CAD build for the part. Positions are in the model's coordinates, mm. A direction names the side the tool comes from. Give positions to 0.01 mm unless a question says otherwise; leave off trailing zeros. Write each loop counter-clockwise with the first axis right and the second up, starting at its lowest first coordinate (ties: lowest second). Pieces come first, ordered by that corner, then holes. Notation, with made-up numbers: (33.5, 45) -> (79.5, 45) arc R15 ccw to (79.5, 57) -> close; hole circle Ø10 at (55, 63.5). An arc over 180 degrees is marked (long way). Use one line per item in the form item = value. Start each with the question number.
Autodesk Inventor part; units mm, degrees
ref_plane "Work Plane1" through (0, 0, 10) normal (0, 0, 1) x (1, 0, 0)
ref_plane "YZ Plane" through (0, 0, 0) normal (1, 0, 0) x (0, 1, 0)
ref_plane "XZ Plane" through (0, 0, 0) normal (0, 1, 0) x (-1, 0, 0)
ref_plane "Work Plane1" through (0, 0, 10) normal (0, 0, 1) x (1, 0, 0)
sketch "Sketch1" plane through (0, 0, 10) normal (0, 0, 1) x (1, 0, 0)
  line L0 (-4.0299, -0.3538) -> (-2.2322, 1.4439) construction
  arc A0 (-1.4439, 2.2322) -> (-2.2322, 1.4439) centre (-0.9299, 0.9299) ccw construction
  line L1 (-1.4439, 2.2322) -> (0.3538, 4.0299) construction
  line L2 (-37.8299, 42.8299) -> (-37.8299, 37.8299) construction
  line L3 (-37.8299, 37.8299) -> (-42.9208, 37.8299) construction
  line L4 (-37.8299, 42.2137) -> (-37.8299, 45.8299) construction
  line L5 (-37.8299, 45.8299) -> (-4.0299, 45.8299) construction
  line L6 (-4.0299, 45.8299) -> (-4.0299, 42.2137) construction
  line L7 (-4.0299, 4.0299) -> (0.3538, 4.0299)
  circle A1 centre (-20.9299, 20.9299) radius 17.5
  line L8 (-20.9299, 58.9723) -> (17.1124, 20.9299) construction
  line L9 (17.1124, 20.9299) -> (-20.9299, -17.1124) construction
  line L10 (-20.9299, -17.1124) -> (-58.9723, 20.9299) construction
  line L11 (-58.9723, 20.9299) -> (-20.9299, 58.9723) construction
  line L12 (-20.9299, 58.9723) -> (-20.9299, -17.1124) construction
  line L13 (17.1124, 20.9299) -> (-58.9723, 20.9299) construction
  line L14 (-20.9299, 58.9723) -> (32.8701, 58.9723) construction
  line L15 (-43.4299, 43.4299) -> (1.5701, 43.4299) construction
  line L16 (1.5701, 43.4299) -> (1.5701, -1.5701) construction
  line L17 (1.5701, -1.5701) -> (-43.4299, -1.5701) construction
  line L18 (-43.4299, -1.5701) -> (-43.4299, 43.4299) construction
  line L19 (-43.4299, 43.4299) -> (1.5701, -1.5701) construction
  line L20 (1.5701, 43.4299) -> (-43.4299, -1.5701) construction
  line L21 (-43.4299, 5.3876) -> (-43.4299, 36.4723)
  line L22 (-43.4299, 36.4723) -> (-36.4723, 43.4299)
  line L23 (-36.4723, 43.4299) -> (-5.3876, 43.4299)
  line L24 (-5.3876, 43.4299) -> (1.5701, 36.4723)
  line L25 (1.5701, 36.4723) -> (1.5701, 5.3876)
  line L26 (1.5701, 5.3876) -> (-5.3876, -1.5701)
  line L27 (-5.3876, -1.5701) -> (-36.4723, -1.5701)
  line L28 (-36.4723, -1.5701) -> (-43.4299, 5.3876)
  line L29 (-4.0299, 42.2137) -> (-37.8299, 42.2137)
  line L30 (-4.0299, -0.3538) -> (-4.0299, 4.0299)
  circle A2 centre (-20.9299, 20.9299) radius 1.5
  line L31 (-10.9299, 10.9299) -> (-30.9299, 10.9299) construction
  line L32 (-30.9299, 10.9299) -> (-30.9299, 30.9299) construction
  line L33 (-30.9299, 30.9299) -> (-10.9299, 30.9299) construction
  line L34 (-10.9299, 30.9299) -> (-10.9299, 10.9299) construction
  line L35 (-10.9299, 10.9299) -> (-30.9299, 30.9299) construction
  line L36 (-30.9299, 10.9299) -> (-10.9299, 30.9299) construction
  circle A3 centre (-30.9299, 30.9299) radius 1.4
  circle A4 centre (-30.9299, 10.9299) radius 1.4
  circle A5 centre (-10.9299, 10.9299) radius 1.4
  line L37 (-45.8299, 37.8299) -> (-42.0723, 37.8299) construction
  line L38 (-42.1723, 37.7299) -> (-45.8299, 37.7299)
  line L39 (-45.8299, 37.7299) -> (-45.8299, 4.1299)
  line L40 (-45.8299, 4.1299) -> (-42.1723, 4.1299)
  line L41 (-42.1723, 4.1299) -> (-42.1723, 37.7299)
  line L42 (-45.8299, 4.0299) -> (-42.0723, 4.0299) construction
  line L43 (-45.8299, 37.8299) -> (-42.0723, 37.8299)
  line L44 (-37.7299, 45.8299) -> (-4.1299, 45.8299)
  line L45 (-4.1299, 45.8299) -> (-4.1299, 42.1723)
  line L46 (-4.1299, 42.1723) -> (-37.7299, 42.1723)
  line L47 (-37.7299, 42.1723) -> (-37.7299, 45.8299)
  line L48 (0.4701, 37.8299) -> (0.4701, 4.0299) construction
  line L49 (0.4701, 4.0299) -> (3.9701, 4.0299) construction
  line L50 (3.9701, 37.8299) -> (3.9701, 4.0299) construction
  line L51 (0.4701, 37.8299) -> (3.9701, 37.8299) construction
  line L52 (-45.8299, -3.9701) -> (-4.0299, -3.9701) construction
  line L53 (0.3124, 37.7299) -> (3.9701, 37.7299)
  line L54 (3.9701, 37.7299) -> (3.9701, 4.1299)
  line L55 (3.9701, 4.1299) -> (0.3124, 4.1299)
  line L56 (0.3124, 4.1299) -> (0.3124, 37.7299)
  line L57 (-4.1713, -0.3538) -> (-37.7299, -0.3538)
  line L58 (-37.7299, -0.3538) -> (-37.7299, -3.9701)
  line L59 (-37.7299, -3.9701) -> (-4.1713, -3.9701)
  line L60 (-4.1713, -3.9701) -> (-4.1713, -0.3538)
  point P0 (-37.8299, 4.0299)
  dimension "d18" = 53.8
  dimension "d19" = 45
  dimension "d20" = 53.8
  dimension "d21" = 45
  dimension "d22" = 45
  dimension "d30" = 20
  dimension "d31" = 20
  dimension "d32" = 2.8
  dimension "d33" = 2.8
  dimension "d34" = 2.8
  dimension "d35" = 3
  dimension "d36" = 0.1
  dimension "d37" = 0.1
  dimension "d38" = 0.1
  dimension "d39" = 0.1
extrude "Extrusion1" add sketch "Sketch1" along normal blind 10 contours L30 L26 L57 L28 L41 L22 L46 L24 L56 L7 | L7 L26 L30 | L56 L24 L25 L26 | L26 L25 L24 L53 L54 L55 | L60 L59 L58 L57 L28 L27 L26 | L26 L27 L28 L57 | L46 L22 L29 L24 | L24 L29 L45 | L40 L39 L38 L22 L21 L28 | L28 L21 L22 L41 | L29 L22 L23 L24 | L24 L23 L22 L29 L47 L44 L45 | L47 L29 L22 | A1 | A2 | A3 | A4 | A5
sketch "Skizze4" plane through (0, 0, 20) normal (0, 0, 1) x (1, 0, 0)
  line L0 (-37.7299, 42.1723) -> (-42.1723, 37.7299)
  line L1 (-42.1723, 37.7299) -> (-45.8299, 37.7299)
  line L2 (-45.8299, 37.7299) -> (-45.8299, 4.1299) construction
  line L3 (-45.8299, 4.1299) -> (-42.1723, 4.1299)
  line L4 (-42.1723, 4.1299) -> (-37.6885, -0.3538)
  line L5 (-37.6885, -0.3538) -> (-37.7299, -0.3538)
  line L6 (-37.7299, -0.3538) -> (-37.7299, -3.9701)
  line L7 (-37.7299, -3.9701) -> (-4.1713, -3.9701) construction
  line L8 (-4.1713, -3.9701) -> (-4.1713, -0.3538)
  line L9 (-4.1713, -0.3538) -> (0.3124, 4.1299)
  line L10 (0.3124, 4.1299) -> (3.9701, 4.1299)
  line L11 (3.9701, 4.1299) -> (3.9701, 37.7299) construction
  line L12 (3.9701, 37.7299) -> (0.3124, 37.7299)
  line L13 (0.3124, 37.7299) -> (-4.1299, 42.1723)
  line L14 (-4.1299, 42.1723) -> (-4.1299, 45.8299)
  line L15 (-4.1299, 45.8299) -> (-37.7299, 45.8299) construction
  line L16 (-37.7299, 45.8299) -> (-37.7299, 42.1723)
  line L17 (-37.9299, 46.0299) -> (-3.9299, 46.0299) construction
  line L18 (-3.9299, 46.0299) -> (-3.9299, 42.2551)
  line L19 (-3.9299, 42.2551) -> (0.3953, 37.9299)
  line L20 (0.3953, 37.9299) -> (4.1701, 37.9299)
  line L21 (4.1701, 37.9299) -> (4.1701, 3.9299) construction
  line L22 (4.1701, 3.9299) -> (0.3953, 3.9299)
  line L23 (0.3953, 3.9299) -> (-3.9713, -0.4367)
  line L24 (-3.9713, -0.4367) -> (-3.9713, -4.1701)
  line L25 (-3.9713, -4.1701) -> (-37.9299, -4.1701) construction
  line L26 (-37.9299, -4.1701) -> (-37.9299, -0.3953)
  line L27 (-37.9299, -0.3953) -> (-42.2551, 3.9299)
  line L28 (-42.2551, 3.9299) -> (-46.0299, 3.9299)
  line L29 (-46.0299, 3.9299) -> (-46.0299, 37.9299) construction
  line L30 (-46.0299, 37.9299) -> (-42.2551, 37.9299)
  line L31 (-42.2551, 37.9299) -> (-37.9299, 42.2551)
  line L32 (-37.9299, 42.2551) -> (-37.9299, 46.0299)
  line L33 (-45.8299, 37.7299) -> (-45.8299, 37.9299)
  line L34 (-4.1299, 45.8299) -> (-37.7299, 45.8299)
  line L35 (-37.7299, 45.8299) -> (-37.9299, 45.8299)
  line L36 (-4.1299, 45.8299) -> (-3.9299, 45.8299)
  line L37 (3.9701, 37.7299) -> (3.9701, 37.9299)
  line L38 (3.9701, 4.1299) -> (3.9701, 37.7299)
  line L39 (3.9701, 4.1299) -> (3.9701, 3.9299)
  line L40 (-4.1713, -3.9701) -> (-3.9713, -3.9701)
  line L41 (-37.7299, -3.9701) -> (-37.9299, -3.9701)
  line L42 (-45.8299, 4.1299) -> (-45.8299, 3.9299)
  point P0 (0, 0)
  dimension "d40" = 0.2
extrude "IM_offset" add sketch "Skizze4" against normal up to surface (10 mm away)
sketch "Sketch25" plane through (0, 0, 10) normal (0, 0, -1) x (-1, 0, 0)
  line L0 (3.9713, -3.9701) -> (37.9299, -3.9701)
  line L1 (37.9299, -3.9701) -> (37.9299, -0.3953)
  line L2 (37.9299, -0.3953) -> (42.2551, 3.9299)
  line L3 (42.2551, 3.9299) -> (45.8299, 3.9299)
  line L4 (45.8299, 3.9299) -> (45.8299, 37.9299)
  line L5 (45.8299, 37.9299) -> (42.2551, 37.9299)
  line L6 (42.2551, 37.9299) -> (37.9299, 42.2551)
  line L7 (37.9299, 42.2551) -> (37.9299, 45.8299)
  line L8 (37.9299, 45.8299) -> (3.9299, 45.8299)
  line L9 (3.9299, 45.8299) -> (3.9299, 42.2551)
  line L10 (3.9299, 42.2551) -> (-0.3953, 37.9299)
  line L11 (-0.3953, 37.9299) -> (-3.9701, 37.9299)
  line L12 (-3.9701, 37.9299) -> (-3.9701, 3.9299)
  line L13 (-3.9701, 3.9299) -> (-0.3953, 3.9299)
  line L14 (-0.3953, 3.9299) -> (3.9713, -0.4367)
  line L15 (3.9713, -0.4367) -> (3.9713, -3.9701)
  circle A0 centre (20.9299, 20.9299) radius 24.9
  circle A1 centre (20.9299, 20.9299) radius 7
  dimension "d167" = 14
extrude "Extrusion21" cut sketch "Sketch25" against normal through all contours A1
sketch "Sketch29" plane through (0, 0, 10) normal (0, 0, -1) x (-1, 0, 0)
  circle A0 centre (38.4299, 30.9299) radius 1
  circle A1 centre (31.9299, 10.4299) radius 1
  circle A2 centre (10.4299, 25.9299) radius 1
  circle A3 centre (31.9299, 10.4299) radius 0.9
  circle A4 centre (38.4299, 30.9299) radius 0.9
  circle A5 centre (10.4299, 25.9299) radius 0.9
  point P0 (0, 0)
  dimension "d171" = 1.8
  dimension "d172" = 1.8
  dimension "d173" = 1.8
extrude "Extrusion23" cut sketch "Sketch29" against normal blind 10 contours A3 | A4 | A5
ref_plane "Arbeitsebene5" through (-37.9299, 20.9299, 10) normal (0, 1, 0) x (1, 0, 0)
ref_plane "Arbeitsebene6" through (-20.9299, 3.9299, 10) normal (1, 0, 0) x (0, 0, -1)
properties part number "20_Cube_Insert_Fiber_STMount_Center"
1) Cut at A-A (x = -15). Give the cut face in (y, z), and give its area (3 significant figures).
2) Wall check: line 1 along X through (y, z) = (10.5, 19.75); line 2 along X through (y, z) = (-0.5, 15.5); line 3 along Y through (x, z) = (-21, 15.5). Give the ranges that are in metal, low to high. Write a range as from..to.
3) Cut at B-B (y = 14.5). Give the cut face in (x, z).
4) Cut at D-D (x = -41). Give the cut face in (y, z) (3 decimals), and give its area (3 significant figures).
5) Cut at C-C (z = 15). Give the cut face in (x, y), and give its area (3 significant figures).
6) 3-axis set-ups, long thin cutter, end or side, ignore diameter. For faces 4 (the face through (-37.93, -2, 15)), 5 (the face through (2, 37.93, 15)), 6 (the face through (2, 3.93, 15)), 7 (the face through (-37.93, 44, 15)): which of +Z, -Z, +X, -X, +Y, -Y reach the whole face in a straight line?
7) Pin check, flat tips, straight feed: pin 1 (4 mm diameter, centred on x = -43, z = 13.5, fed in from -Y); pin 2 (1.1 mm diameter, centred on y = 45, z = 16.5, fed in from -X); pin 3 (1.8 mm diameter, centred on y = 44, z = 17.5, fed in from +X). Stop position of each tip, or through.
8) Two-plate mould, pull along Y, no slides. Class faces 1 (the face through (-24.693, 26.832, 14.93)), 2 (the face through (-40.123, 40.062, 15.07)), 3 (the face through (-3.93, 44, 15)): released by +Y, released by -Y, zero draft, split by the parting line, or undercut.
Final values:
q1.outline = (-3.97, 10) -> (17.21, 10) -> (17.21, 20) -> (-3.97, 20) -> close; (24.65, 10) -> (45.83, 10) -> (45.83, 20) -> (24.65, 20) -> close
q1.area = 424 mm^2
q2.line_1 = -45.83..-32.83, -31.03..3.97
q2.line_2 = -37.93..-3.97
q2.line_3 = -3.97..13.93, 27.93..45.83
q3.outline = (-45.83, 10) -> (-23.7, 10) -> (-23.7, 20) -> (-45.83, 20) -> close; (-18.16, 10) -> (3.97, 10) -> (3.97, 20) -> (-18.16, 20) -> close
q4.outline = (2.675, 10) -> (39.185, 10) -> (39.185, 20) -> (2.675, 20) -> close
q4.area = 365 mm^2
q5.outline = (-45.83, 3.93) -> (-42.26, 3.93) -> (-37.93, -0.4) -> (-37.93, -3.97) -> (-3.97, -3.97) -> (-3.97, -0.44) -> (0.4, 3.93) -> (3.97, 3.93) -> (3.97, 37.93) -> (0.4, 37.93) -> (-3.93, 42.26) -> (-3.93, 45.83) -> (-37.93, 45.83) -> (-37.93, 42.26) -> (-42.26, 37.93) -> (-45.83, 37.93) -> close; hole circle Ø1.8 at (-38.43, 30.93); hole circle Ø1.8 at (-31.93, 10.43); hole circle Ø14 at (-20.93, 20.93); hole circle Ø1.8 at (-10.43, 25.93)
q5.area = 2,110 mm^2
q6.face_4 = +Z, -Z, -X, -Y
q6.face_5 = +Z, -Z, +X, +Y
q6.face_6 = +Z, -Z, +X, -Y
q6.face_7 = +Z, -Z, -X, +Y
q7.pin_1 = 2.67
q7.pin_2 = -37.93
q7.pin_3 = -3.93
q8.face_1 = undercut
q8.face_2 = released by +Y
q8.face_3 = zero draft
